from build123d import *

# Parameters (mm, degrees)
SKETCH1_W           = 6.5
SKETCH1_H           = 13
BOSS_EXTRUDE1_DEPTH = 3
SKETCH4_R           = 1.025
CUT_EXTRUDE1_DEPTH  = 7
EXTRUDE_THIN1_DEPTH = 1.85


with BuildPart() as part:
    # Sketch1 → Boss-Extrude1 (new body, symmetric)
    with BuildSketch(Plane.XY):
        Rectangle(SKETCH1_W, SKETCH1_H)
    extrude(amount=BOSS_EXTRUDE1_DEPTH, both=True)

    # Sketch4 → Cut-Extrude1 (cut, through all)
    with BuildSketch(Plane.XY.offset(3)):
        with Locations((1.75, 3.25)):
            Circle(SKETCH4_R)
        with Locations((1.75, -3.25)):
            Circle(SKETCH4_R)
    extrude(amount=-CUT_EXTRUDE1_DEPTH, mode=Mode.SUBTRACT)

    # Sketch9 → Extrude-Thin1 (add, symmetric)
    with BuildSketch(Plane.XY):
        with BuildLine():
            Line((-3.25, 5.375), (-3.75, 5.375))
            Line((-3.75, 5.375), (-5.25, -2.991600265))
            ThreePointArc((-5.25, -2.991600265), (-8.44213538, -5.21314741), (-6.220588235, -8.40528279))
            Line((-6.220588235, -8.40528279), (-6.264705882, -8.651359268))
            ThreePointArc((-6.264705882, -8.651359268), (-8.707721009, -5.292635692), (-5.453800269, -2.711677189))
            Line((-5.453800269, -2.711677189), (-3.959165007, 5.625))
            Line((-3.959165007, 5.625), (-3.25, 5.625))
            Line((-3.25, 5.625), (-3.25, 5.375))
        make_face()
    extrude(amount=EXTRUDE_THIN1_DEPTH, both=True)


solid = part.part
Input: part model. Units: mm. Frame: model coordinates. A direction names the side the tool comes from. Coordinates: 2 decimals unless noted, no trailing zeros. Loops run counter-clockwise (first coordinate to the right, second up) from the corner with the lowest first, then second, coordinate; pieces in that order, holes last.
(1) Section D-D on x = -7. Return the cut outline in (y, z).
(2) Section A-A on z = 0.15. Return the cut outline in (x, y) (3 decimals), then the cut area to 3 significant figures.
(3) Section C-C on y = 2. Return the cut outline in (x, z), then the cut area to 3 significant figures.
(4) First-contact query: pin 1 Ø2 at (y, z) = (0.5, 1.5) entering from -X; pin 2 Ø3 at (x, y) = (-6.5, -4) entering from +Z; pin 3 Ø1.2 at (x, y) = (1.75, 3.25) entering from -Z; pin 4 Ø1.8 at (x, z) = (-0.5, -0.5) entering from -Y. Flat tips, straight axial feed; report the tip coordinate or a pass-through.
(5) Set-up query: faces 4 (the face through (-4.49, 1.25, 0.03)), 5 (the face through (0, -6.5, 0)), 6 (the face through (-8.43, -5.15, 0.03)). Return all of +Z, -Z, +X, -X, +Y, -Y with unobstructed straight access to the full face (end or side cutting, diameter ignored); none if empty.
(6) Pull-direction query (X, two-part tool) for faces 1 (the face through (0, 0, 3)), 2 (the face through (3.25, 0, 0)), 3 (the face through (0.937, 2.626, 0.042)); classes: released by +X, released by -X, zero draft, split by the parting line, or undercut.
(7) Material intervals for probe 1 along Y at (x, z) = (1.75, -1.5) (3 decimals); probe 2 along X at (y, z) = (4, -1.3); probe 3 along Y at (x, z) = (2.5, 1.3), sorted ascending.
(8) Section B-B on x = 1.75. Return the cut outline in (y, z) (3 decimals), then the cut area to 3 significant figures.
Data:
1. outline: (-8.42, -1.85) - (-8.14, -1.85) - (-8.14, 1.85) - (-8.42, 1.85) - close; (-3.26, -1.85) - (-2.98, -1.85) - (-2.98, 1.85) - (-3.26, 1.85) - close
2. outline: (-6.265, -8.651) - (-6.221, -8.405) arc R2.75 cw to (-5.25, -2.992) - (-3.75, 5.375) - (-3.25, 5.375) - (-3.25, -6.5) - (3.25, -6.5) - (3.25, 6.5) - (-3.25, 6.5) - (-3.25, 5.625) - (-3.959, 5.625) - (-5.454, -2.712) arc R3 ccw to start; hole circle Ø2.05 at (1.75, -3.25); hole circle Ø2.05 at (1.75, 3.25)
2. area: 82.4 mm2
3. outline: (-4.61, -1.85) - (-4.36, -1.85) - (-4.36, 1.85) - (-4.61, 1.85) - close; (-3.25, -3) - (3.25, -3) - (3.25, 3) - (-3.25, 3) - close
3. area: 39.9 mm2
4. pin 1: stops at x = -5.06
4. pin 2: stops at z = 1.85
4. pin 3: passes through
4. pin 4: stops at y = -6.5
5. face 4: +Z, -Z, -Y
5. face 5: +Z, -Z, +X, -Y
5. face 6: +Z, -Z
6. face 1: zero draft
6. face 2: released by +X
6. face 3: undercut
7. probe 1: y = -6.5 to -4.275, -2.225 to 2.225, 4.275 to 6.5
7. probe 2: x = -4.25 to -4, -3.25 to 1.05, 2.45 to 3.25
7. probe 3: y = -6.5 to -3.95, -2.55 to 2.55, 3.95 to 6.5
8. outline: (-6.5, -3) - (-4.275, -3) - (-4.275, 3) - (-6.5, 3) - close; (-2.225, -3) - (2.225, -3) - (2.225, 3) - (-2.225, 3) - close; (4.275, -3) - (6.5, -3) - (6.5, 3) - (4.275, 3) - close
8. area: 53.4 mm2
